```python
from build123d import *

# Parameters (mm, degrees)
BOSS_EXTRU_1_DEPTH           = 2.5
ENL_V_MAT_EXTRU_1_REACH      = 169.131
ESQUISSE3_R                  = 1.75
BOSS_EXTRU_2_DEPTH           = 10
BOSS_EXTRU_2_DRAFT           = -3
ESQUISSE4_W                  = 32.5
ESQUISSE4_H                  = 2.5
BOSS_EXTRU_2_PROFILE_2_DEPTH = 10
BOSS_EXTRU_2_PROFILE_2_DRAFT = -3
ENL_V_MAT_EXTRU_2_REACH      = 200.265
ESQUISSE8_R                  = 1
BOSS_EXTRU_3_REACH           = 200.265
ESQUISSE9_R                  = 3.5
ESQUISSE9_R_2                = 1


with BuildPart() as part:
    # Esquisse1 → Boss.-Extru.1 (new body)
    with BuildSketch(Plane.XY):
        with BuildLine():
            Line((149.100058284, 75.46875), (-12.711143092, 75.46875))
            ThreePointArc((-12.711143092, 75.46875), (-20.816828901, 74.638864342), (-28.58617509, 72.183642878))
            Line((-28.58617509, 72.183642878), (-102.884320715, 40.05811161))
            ThreePointArc((-102.884320715, 40.05811161), (-105.899941716, 35.46875), (-102.884320715, 30.87938839))
            Line((-102.884320715, 30.87938839), (-28.58617509, -1.246142878))
            ThreePointArc((-28.58617509, -1.246142878), (-20.816828901, -3.701364342), (-12.711143092, -4.53125))
            Line((-12.711143092, -4.53125), (149.100058284, -4.53125))
            Line((149.100058284, -4.53125), (149.100058284, 75.46875))
        make_face()
    extrude(amount=BOSS_EXTRU_1_DEPTH)

    # Esquisse3 → Enlèv. mat.-Extru.1 (cut, up to next)
    with BuildSketch(Plane.XY.offset(2.5), mode=Mode.PRIVATE) as enl_v_mat_extru_1_sk1:
        with Locations((97.100058284, 44.46875)):
            Circle(ESQUISSE3_R)
    enl_v_mat_extru_1_tool1 = extrude(enl_v_mat_extru_1_sk1.sketch, amount=-ENL_V_MAT_EXTRU_1_REACH, mode=Mode.PRIVATE) & part.part
    # Esquisse3 → Enlèv. mat.-Extru.1 (cut, up to next)
    with BuildSketch(Plane.XY.offset(2.5), mode=Mode.PRIVATE) as enl_v_mat_extru_1_sk2:
        with Locations((97.100058284, 26.46875)):
            Circle(ESQUISSE3_R)
    enl_v_mat_extru_1_tool2 = extrude(enl_v_mat_extru_1_sk2.sketch, amount=-ENL_V_MAT_EXTRU_1_REACH, mode=Mode.PRIVATE) & part.part
    # Esquisse3 → Enlèv. mat.-Extru.1 (cut, up to next)
    with BuildSketch(Plane.XY.offset(2.5), mode=Mode.PRIVATE) as enl_v_mat_extru_1_sk3:
        with Locations((109.100058284, 26.46875)):
            Circle(ESQUISSE3_R)
    enl_v_mat_extru_1_tool3 = extrude(enl_v_mat_extru_1_sk3.sketch, amount=-ENL_V_MAT_EXTRU_1_REACH, mode=Mode.PRIVATE) & part.part
    # Esquisse3 → Enlèv. mat.-Extru.1 (cut, up to next)
    with BuildSketch(Plane.XY.offset(2.5), mode=Mode.PRIVATE) as enl_v_mat_extru_1_sk4:
        with Locations((109.100058284, 44.46875)):
            Circle(ESQUISSE3_R)
    enl_v_mat_extru_1_tool4 = extrude(enl_v_mat_extru_1_sk4.sketch, amount=-ENL_V_MAT_EXTRU_1_REACH, mode=Mode.PRIVATE) & part.part
    add(enl_v_mat_extru_1_tool1.solids().sort_by_distance((97.100058, 44.46875, 2.5))[0], mode=Mode.SUBTRACT)
    add(enl_v_mat_extru_1_tool2.solids().sort_by_distance((97.100058, 26.46875, 2.5))[0], mode=Mode.SUBTRACT)
    add(enl_v_mat_extru_1_tool3.solids().sort_by_distance((109.100058, 26.46875, 2.5))[0], mode=Mode.SUBTRACT)
    add(enl_v_mat_extru_1_tool4.solids().sort_by_distance((109.100058, 44.46875, 2.5))[0], mode=Mode.SUBTRACT)


with BuildPart() as boss_extru_2_tool:
    # Esquisse4 → Boss.-Extru.2 (with draft: the straight prism first)
    with BuildSketch(Plane(origin=(0, 0, 2.5), x_dir=(-1, 0, 0), z_dir=(0, 0, -1))):
        Polygon((-51.600058284, 0.96875), (-89.100058284, 0.96875), (-89.100058284, 67.46875), (-91.600058284, 67.46875), (-91.600058284, -1.53125), (-49.100058284, -1.53125), (-49.100058284, 67.46875), (-51.600058284, 67.46875), align=None)
    extrude(amount=-BOSS_EXTRU_2_DEPTH)
    # Boss.-Extru.2: the draft: its side faces are tilted about the plane it starts from
    boss_extru_2_sides = [boss_extru_2_tool.faces().sort_by_distance(p)[0] for p in [
        (70.350058284, 0.96875, 7.5),
        (89.100058284, 34.21875, 7.5),
        (90.350058284, 67.46875, 7.5),
        (91.600058284, 32.96875, 7.5),
        (70.350058284, -1.53125, 7.5),
        (49.100058284, 32.96875, 7.5),
        (50.350058284, 67.46875, 7.5),
        (51.600058284, 34.21875, 7.5),
    ]]
    draft(boss_extru_2_sides, Plane(origin=(0, 0, 2.5), x_dir=(-1, 0, 0), z_dir=(0, 0, -1)), BOSS_EXTRU_2_DRAFT)


with BuildPart() as part_1:
    add(part.part)

    # Boss.-Extru.2: add boss_extru_2_tool
    add(boss_extru_2_tool.part)


with BuildPart() as boss_extru_2_profile_2_tool:
    # Esquisse4 → Boss.-Extru.2 profile 2 (with draft: the straight prism first)
    with BuildSketch(Plane(origin=(0, 0, 2.5), x_dir=(-1, 0, 0), z_dir=(0, 0, -1))):
        with Locations((-70.350058284, 71.21875)):
            Rectangle(ESQUISSE4_W, ESQUISSE4_H)
    extrude(amount=-BOSS_EXTRU_2_PROFILE_2_DEPTH)
    # Boss.-Extru.2 profile 2: the draft: its side faces are tilted about the plane it starts from
    boss_extru_2_profile_2_sides = [boss_extru_2_profile_2_tool.faces().sort_by_distance(p)[0] for p in [
        (54.100058284, 71.21875, 7.5),
        (70.350058284, 72.46875, 7.5),
        (86.600058284, 71.21875, 7.5),
        (70.350058284, 69.96875, 7.5),
    ]]
    draft(boss_extru_2_profile_2_sides, Plane(origin=(0, 0, 2.5), x_dir=(-1, 0, 0), z_dir=(0, 0, -1)), BOSS_EXTRU_2_PROFILE_2_DRAFT)


with BuildPart() as part_2:
    add(part_1.part)

    # Boss.-Extru.2 profile 2: add boss_extru_2_profile_2_tool
    add(boss_extru_2_profile_2_tool.part)

    # Balayage1: sweep along a path in Esquisse5
    with BuildLine(Plane.XY.offset(2.5)) as balayage1_path:
        Line((149.100058284, 75.46875), (-12.711143092, 75.46875))
        ThreePointArc((-12.711143092, 75.46875), (-20.816828901, 74.638864342), (-28.58617509, 72.183642878))
        Line((-28.58617509, 72.183642878), (-102.884320715, 40.05811161))
        ThreePointArc((-102.884320715, 40.05811161), (-105.899941716, 35.46875), (-102.884320715, 30.87938839))
        Line((-102.884320715, 30.87938839), (-28.58617509, -1.246142878))
        ThreePointArc((-28.58617509, -1.246142878), (-20.816828901, -3.701364342), (-12.711143092, -4.53125))
        Line((-12.711143092, -4.53125), (149.100058284, -4.53125))
        Line((149.100058284, -4.53125), (149.100058284, 75.46875))
    # Esquisse7 → Balayage1 (sweep)
    with BuildSketch(Plane(origin=(149.100058284, 0, 0), x_dir=(0, 0, -1), z_dir=(1, 0, 0))):
        with BuildLine():
            Line((-2.5, 75.46875), (0, 75.46875))
            add(Edge.make_bspline(
                [(0, 75.46875), (0, 86.411621691), (-9.099638508, 95.407035507), (-40, 95.46875)],
                knots=[0, 0, 0, 0, 1, 1, 1, 1], degree=3))
            Line((-40, 95.46875), (-40, 92.96875))
            add(Edge.make_bspline(
                [(-40, 92.96875), (-36.824934583, 92.96875), (-2.5, 94.513588254), (-2.5, 75.46875)],
                knots=[0, 0, 0, 0, 1, 1, 1, 1], degree=3))
        make_face()
    sweep(path=balayage1_path.line, transition=Transition.RIGHT)

    # Esquisse8 → Enlèv. mat.-Extru.2 (cut, up to next)
    with BuildSketch(Plane(origin=(0, 0, 0), x_dir=(-1, 0, 0), z_dir=(0, 0, -1)), mode=Mode.PRIVATE) as enl_v_mat_extru_2_sk1:
        with Locations((-154.100058284, 55.46875)):
            Circle(ESQUISSE8_R)
    enl_v_mat_extru_2_tool1 = extrude(enl_v_mat_extru_2_sk1.sketch, amount=-ENL_V_MAT_EXTRU_2_REACH, mode=Mode.PRIVATE) & part_2.part
    # Esquisse8 → Enlèv. mat.-Extru.2 (cut, up to next)
    with BuildSketch(Plane(origin=(0, 0, 0), x_dir=(-1, 0, 0), z_dir=(0, 0, -1)), mode=Mode.PRIVATE) as enl_v_mat_extru_2_sk2:
        with Locations((-154.100058284, 15.46875)):
            Circle(ESQUISSE8_R)
    enl_v_mat_extru_2_tool2 = extrude(enl_v_mat_extru_2_sk2.sketch, amount=-ENL_V_MAT_EXTRU_2_REACH, mode=Mode.PRIVATE) & part_2.part
    add(enl_v_mat_extru_2_tool1.solids().sort_by_distance((154.100058, 55.46875, 0))[0], mode=Mode.SUBTRACT)
    add(enl_v_mat_extru_2_tool2.solids().sort_by_distance((154.100058, 15.46875, 0))[0], mode=Mode.SUBTRACT)

    # Esquisse9 → Boss.-Extru.3 (add, up to next)
    with BuildSketch(Plane.XY.offset(40), mode=Mode.PRIVATE) as boss_extru_3_sk1:
        with Locations((154.100058284, 15.46875)):
            Circle(ESQUISSE9_R)
        with Locations(Location((154.100058284, 15.46875, 0), (0, 0, 180))):
            Circle(ESQUISSE9_R_2, mode=Mode.SUBTRACT)
    boss_extru_3_tool1 = extrude(boss_extru_3_sk1.sketch, amount=-BOSS_EXTRU_3_REACH, mode=Mode.PRIVATE) - part_2.part
    # Esquisse9 → Boss.-Extru.3 (add, up to next)
    with BuildSketch(Plane.XY.offset(40), mode=Mode.PRIVATE) as boss_extru_3_sk2:
        with Locations((154.100058284, 55.46875)):
            Circle(ESQUISSE9_R)
        with Locations(Location((154.100058284, 55.46875, 0), (0, 0, 180))):
            Circle(ESQUISSE9_R_2, mode=Mode.SUBTRACT)
    boss_extru_3_tool2 = extrude(boss_extru_3_sk2.sketch, amount=-BOSS_EXTRU_3_REACH, mode=Mode.PRIVATE) - part_2.part
    add(boss_extru_3_tool1.solids().sort_by_distance((150.699053, 15.46875, 40))[0])
    add(boss_extru_3_tool2.solids().sort_by_distance((150.699053, 55.46875, 40))[0])


solid = part_2.part
```
Part model, mm, in its own coordinate system. A direction names the side the tool comes from. Round coordinates to 2 decimals unless told otherwise and drop trailing zeros. Use a Markdown table: item, result.
1) Tool access for faces 1 (the cylindrical face through (150.603, 55.623, 21.549)), 2 (the flat face through (153, 15, 40)): list every direction of +Z, -Z, +X, -X, +Y, -Y with a clear straight run to the whole face (end or side of a thin tool).
The answers:
| item | result |
|---|---|
| face 1 | +Z |
| face 2 | +Z, +X, -X, +Y, -Y |
2) Cut at A-A, the plane z = 35.5. State how many separate pieces and enclosed holes the cut face has, and give its area (3 significant figures).
The answers:
| item | result |
|---|---|
| separate pieces | 3 |
| enclosed holes | 3 |
| area | 1,860 mm2 |
3) Drop flat-ended pins along their axis: pin 1 Ø1 at (x, z) = (62, 10) entering from +Y; pin 2 Ø1.2 at (x, y) = (154.1, 55.47) entering from +Z; pin 3 Ø5 at (y, z) = (25, 33.5) entering from -X; pin 4 Ø6 at (x, z) = (60.5, 23.5) entering from -Y. Give the stop position or say it passes through.
The answers:
| item | result |
|---|---|
| pin 1 | stops at y = 90.66 |
| pin 2 | passes through |
| pin 3 | stops at x = -124.44 |
| pin 4 | stops at y = -23.81 |
4) Pull direction X, two halves, no side cores. Call faces 3 (the flat face through (91.34, 33.45, 7.43)), 4 (the flat face through (48, 36, 0)), 5 (the flat face through (70.578, 70.227, 7.43)): pulls with the +X half, pulls with the -X half, needs draft (parallel to the pull), parting line crosses it, or undercut.
The answers:
| item | result |
|---|---|
| face 3 | undercut |
| face 4 | needs draft |
| face 5 | undercut |
5) Probe line 1 (X direction, y = 52.5, z = 8); line 2 (X direction, y = 57, z = 19); line 3 (Y direction, x = 153.5, z = 9.5). List the from-to ranges inside material, lowest first. Write a range as [from, to].
The answers:
| item | result |
|---|---|
| line 1 | x = [-108.93, -101.41], [49.39, 51.31], [89.39, 91.31], [152.25, 155.95], [159.94, 162.93] |
| line 2 | x = [-109.12, -103.12], [150.95, 157.25], [164.74, 167.12] |
| line 3 | y = [-19.22, -16.41], [12.02, 14.67], [16.27, 18.92], [52.02, 54.67], [56.27, 58.92], [87.34, 90.16] |
